Check sheet for the modelled part. Datum: model origin and axes. Units: mm. A direction names the side the tool comes from. Give positions to 0.01 mm unless a question says otherwise; leave off trailing zeros. Order: outer loops, then holes, each group sorted by start corner. A loop starts at its lowest first (then second) coordinate and runs counter-clockwise, first axis right, second up. Notation, with made-up numbers: (54, 77) -> (83, 77) arc R20 ccw to (83, 110) -> close; hole circle Ø4 at (51.5, 69). An arc over 180 degrees is marked (long way). Answer in a Markdown table with one row per item. Add a question column.
(1) Go/stop test with flat-tipped pins: pin 1 (2 mm diameter, centred on x = 96, y = -109.5, fed in from -Z); pin 2 (3 mm diameter, centred on x = -118, y = 39, fed in from -Z); pin 3 (1.5 mm diameter, centred on x = -21.5, y = 115.5, fed in from -Z); pin 4 (3 mm diameter, centred on x = -89.5, z = 1, fed in from -Y). Record where each tip stops, or that it passes through.
(2) Cross-section at A-A (y = 0). Record the cut outline in (x, z), then the cut area to 3 significant figures.
(3) Thickness scan on L1, parallel to Y at x = 0, z = 5.5; L2, parallel to X at y = 0, z = 1.1; L3, parallel to Z at x = -64.5, y = 121. Record the ranges inside material, lowest first. Write a range as [from, to].
(4) Set-up check for faces 4 (the face through (8.172, 154.888, 9.715)), 5 (the face through (138.513, -70.289, 4.437)), 6 (the face through (88.2, -109, 0)), 7 (the face through (-138.47, -70.13, 4.44)), 8 (the face through (-82, 94, 5)): record each of +Z, -Z, +X, -X, +Y, -Y from which the full face is reachable in a straight line by a thin tool's end or side.
(5) Release check for a two-part mould opening along X. For faces 1 (the face through (0, 161, 4)), 2 (the face through (-119.884, 5.276, 7.465)), 3 (the face through (-8.385, 155.1, 4.437)) record: released by +X, released by -X, zero draft, split by the parting line, or undercut.
```python
from build123d import *
from build123d.topology import SkipClean

# Parameters (mm, degrees)
SKETCH1_R                = 150
SKETCH1_R_2              = 140
BOSS_EXTRUDE1_DEPTH      = 5
SKETCH2_R                = 150
SKETCH2_R_2              = 120
BOSS_EXTRUDE2_DEPTH      = 5
BOSS_EXTRUDE3_START      = -10
SKETCH3_R                = 2.65
BOSS_EXTRUDE3_DEPTH      = 10
FILLET1_R                = 6
CIRPATTERN1_COUNT        = 3
FILLET1_OF_CIRPATTERN1_R = 6
FILLET2_R                = 1
CUT_EXTRUDE2_DEPTH       = 5
FILLET3_R                = 2.5


with BuildPart() as part:
    # Sketch1 → Boss-Extrude1 (new body)
    with BuildSketch(Plane.XY):
        Circle(SKETCH1_R)
        Circle(SKETCH1_R_2, mode=Mode.SUBTRACT)
    extrude(amount=BOSS_EXTRUDE1_DEPTH)

    # Sketch2 → Boss-Extrude2 (add)
    with BuildSketch(Plane.XY.offset(5)):
        Circle(SKETCH2_R)
        Circle(SKETCH2_R_2, mode=Mode.SUBTRACT)
    extrude(amount=BOSS_EXTRUDE2_DEPTH)

    # Sketch3 → Boss-Extrude3 (add)
    with BuildSketch(Plane.XY.offset(10).offset(BOSS_EXTRUDE3_START)):
        with BuildLine():
            ThreePointArc((-14.154618867, 149.330662507), (0, 150), (14.154618867, 149.330662507))
            Line((14.154618867, 149.330662507), (4.242640687, 159.242640687))
            ThreePointArc((4.242640687, 159.242640687), (0, 161), (-4.242640687, 159.242640687))
            Line((-4.242640687, 159.242640687), (-14.154618867, 149.330662507))
        make_face()
        with Locations((0, 155)):
            Circle(SKETCH3_R, mode=Mode.SUBTRACT)
    boss_extrude3 = extrude(amount=BOSS_EXTRUDE3_DEPTH)

    # Fillet1
    fillet1_edges = [part.edges().sort_by_distance(p)[0] for p in [
        (-14.154618867, 149.330662507, 5),
        (14.154618867, 149.330662507, 5),
    ]]
    fillet(fillet1_edges, radius=FILLET1_R)

    # CirPattern1: Boss-Extrude3 ×3 about axis
    cirpattern1_axis = Axis((0, 0, 0), (0, 0, 1))
    for i in range(1, CIRPATTERN1_COUNT):
        add(boss_extrude3.rotate(cirpattern1_axis, i * 360 / CIRPATTERN1_COUNT))

    # Fillet1 of CirPattern1
    fillet1_of_cirpattern1_edges = [part.edges().sort_by_distance(p)[0] for p in [
        (-122.246837861, -86.923590773, 5),
        (-136.401456729, -62.407071733, 5),
        (136.401456729, -62.407071733, 5),
        (122.246837861, -86.923590773, 5),
    ]]
    fillet(fillet1_of_cirpattern1_edges, radius=FILLET1_OF_CIRPATTERN1_R)

    # Fillet2
    fillet2_edges = [part.edges().sort_by_distance(p)[0] for p in [
        (8.443648708, 155.041632666, 10),
        (0, 161, 10),
        (-8.443648708, 155.041632666, 10),
        (-129.903810568, 75, 10),
        (-14.29409564, 149.672599518, 10),
        (14.29409564, 149.672599518, 10),
        (-138.491816887, -70.208402051, 10),
        (-139.430090009, -80.5, 10),
        (-130.048168179, -84.833230615, 10),
        (130.048168179, -84.833230615, 10),
        (139.430090009, -80.5, 10),
        (138.491816887, -70.208402051, 10),
        (0, -150, 10),
        (-122.473225614, -87.215349707, 10),
        (-136.767321253, -62.457249811, 10),
        (129.903810568, 75, 10),
        (136.767321253, -62.457249811, 10),
        (122.473225614, -87.215349707, 10),
    ]]
    fillet(fillet2_edges, radius=FILLET2_R)

    # Sketch4 → Cut-Extrude2 (cut)
    with SkipClean():  # the faces are left unmerged after this step: merging them gives an invalid solid
        with BuildSketch(Plane(origin=(0, 0, 0), x_dir=(-1, 0, 0), z_dir=(0, 0, -1))):
            with BuildLine():
                ThreePointArc((57.604193668, 127.599987743), (88.666685349, 108.343061196), (113.686688952, 81.702734074))
                Line((113.686688952, 81.702734074), (121.807166734, 87.538643651))
                ThreePointArc((121.807166734, 87.538643651), (95.000020016, 116.081851281), (61.718778929, 136.714272581))
                Line((61.718778929, 136.714272581), (57.604193668, 127.599987743))
            make_face()
            with BuildLine():
                ThreePointArc((55.546901037, 123.042845323), (85.500018015, 104.473666153), (109.626450061, 78.784779286))
                Line((109.626450061, 78.784779286), (113.686688952, 81.702734074))
                ThreePointArc((113.686688952, 81.702734074), (88.666685349, 108.343061196), (57.604193668, 127.599987743))
                Line((57.604193668, 127.599987743), (55.546901037, 123.042845323))
            make_face()
            with BuildLine():
                Line((113.686688952, 81.702734074), (109.626450061, 78.784779286))
                ThreePointArc((109.626450061, 78.784779286), (128.500137662, 41.384956456), (135, 0))
                ThreePointArc((135, 0), (-113.410386738, -73.233081186), (55.546901037, 123.042845323))
                Line((55.546901037, 123.042845323), (57.604193668, 127.599987743))
                ThreePointArc((57.604193668, 127.599987743), (-117.610771432, -75.945417526), (140, 0))
                ThreePointArc((140, 0), (133.25940202, 42.917732621), (113.686688952, 81.702734074))
            make_face()
        extrude(amount=-CUT_EXTRUDE2_DEPTH, mode=Mode.SUBTRACT)

    # Fillet3
    # the kernel refuses this fillet: 2.5 mm, written as the material it adds along each edge
    with BuildSketch(Plane(origin=(-55.032577879, 121.903559718, 5), x_dir=(0, 0, -1), z_dir=(-0.41145852619651707, 0.9114284838758278, 0))) as fillet3_piece_1_section:
        with BuildLine():
            CenterArc((FILLET3_R, FILLET3_R), FILLET3_R, 180, 90)
            Line((0, FILLET3_R), (0, 0))
            Line((0, 0), (FILLET3_R, 0))
        make_face()
    fillet3_piece_1 = extrude(amount=22.5, mode=Mode.PRIVATE)
    fillet3_piece_1 = fillet3_piece_1 & Plane(origin=(0, 0, 4.434016132), x_dir=(1, 0, 0), z_dir=(0, 0, -1)) * Cylinder(150, 56, mode=Mode.PRIVATE)
    fillet3_piece_1 = fillet3_piece_1 - Plane(origin=(0, 0, 4.434016132), x_dir=(1, 0, 0), z_dir=(0, 0, -1)) * Cylinder(140, 56, mode=Mode.PRIVATE)
    add(fillet3_piece_1)
    with BuildSketch(Plane(origin=(-108.611390338, 78.055290588, 5), x_dir=(0, 0, -1), z_dir=(-0.8120477782278018, 0.5835909576709453, 0))) as fillet3_piece_2_section:
        with BuildLine():
            CenterArc((FILLET3_R, -FILLET3_R), FILLET3_R, 90, 90)
            Line((0, -FILLET3_R), (0, 0))
            Line((0, 0), (FILLET3_R, 0))
        make_face()
    fillet3_piece_2 = extrude(amount=22.5, mode=Mode.PRIVATE)
    fillet3_piece_2 = fillet3_piece_2 & Plane(origin=(0, 0, 4.434018279), x_dir=(1, 0, 0), z_dir=(0, 0, -1)) * Cylinder(150, 55, mode=Mode.PRIVATE)
    fillet3_piece_2 = fillet3_piece_2 - Plane(origin=(0, 0, 4.434018279), x_dir=(-0.41145852619650086, 0.9114284838758352, 0), z_dir=(0, 0, -1)) * Cylinder(140, 55, mode=Mode.PRIVATE)
    add(fillet3_piece_2)
    # the kernel refuses this fillet: 2.5 mm, written as the material it takes off along each edge
    with BuildSketch(Plane(origin=(-64.290394718, 142.410700606, 0), x_dir=(0.9114284838758278, 0.4114585261965171, 0), z_dir=(0.41145852619651707, -0.9114284838758278, 0))) as fillet3_2_piece_1:
        with BuildLine():
            CenterArc((FILLET3_R, FILLET3_R), FILLET3_R, 180, 90)
            Line((0, FILLET3_R), (0, 0))
            Line((0, 0), (FILLET3_R, 0))
        make_face()
    extrude(amount=22.5, mode=Mode.SUBTRACT)
    with BuildSketch(Plane(origin=(-126.882465348, 91.186087136, 0), x_dir=(-0.5835909576709452, -0.8120477782278016, 0), z_dir=(0.8120477782278018, -0.5835909576709453, 0))) as fillet3_2_piece_2:
        with BuildLine():
            CenterArc((FILLET3_R, -FILLET3_R), FILLET3_R, 90, 90)
            Line((0, -FILLET3_R), (0, 0))
            Line((0, 0), (FILLET3_R, 0))
        make_face()
    extrude(amount=22.5, mode=Mode.SUBTRACT)


solid = part.part
```
Answer below:
| question | item | result |
|---|---|---|
| 1 | pin 1 | stops at z = 0 |
| 1 | pin 2 | stops at z = 5 |
| 1 | pin 3 | passes through |
| 1 | pin 4 | stops at y = -121.47 |
| 2 | outline | (-150, 0) -> (-140, 0) -> (-140, 5) -> (-120, 5) -> (-120, 10) -> (-149, 10) arc R1 ccw to (-150, 9) -> close; (120, 5) -> (140, 5) -> (140, 0) -> (150, 0) -> (150, 9) arc R1 ccw to (149, 10) -> (120, 10) -> close |
| 2 | area | 400 mm² |
| 3 | L1 | y = [-150, -120], [120, 152.35], [157.65, 161] |
| 3 | L2 | x = [-150, -140], [140, 150] |
| 3 | L3 | z = [5, 10] |
| 4 | face 4 | +Z, +X, +Y |
| 4 | face 5 | +Z, -Z, +X |
| 4 | face 6 | -Z, +X, -X, +Y, -Y |
| 4 | face 7 | +Z, -Z, -X |
| 4 | face 8 | -Z |
| 5 | face 1 | split by the parting line |
| 5 | face 2 | undercut |
| 5 | face 3 | released by -X |
